Can you work these out from the model? Positions are in its coordinate system, mm. A direction names the side the tool comes from. Coordinates: 2 decimals unless noted, no trailing zeros. Write each loop counter-clockwise with the first axis right and the second up, starting at its lowest first coordinate (ties: lowest second). Pieces come first, ordered by that corner, then holes. Notation, with made-up numbers: (-33, 34) - (22, 34) arc R26 cw to (22, 51) - close; hole circle Ø7 at (1.25, 9). An arc over 180 degrees is marked (long way). Write each question's results on one line, items separated by ' | '. Start each with the question number.
```python
from build123d import *

# Parameters (mm, degrees)
SKETCH_1_W                = 120
SKETCH_1_H                = 20
EXTRUDE_1_DEPTH           = 4
HOLE_WIZARD_1_D           = 5.5
HOLE_WIZARD_1_CBORE_D     = 9.4
HOLE_WIZARD_1_CBORE_DEPTH = 5
HOLE_WIZARD_M5_2_D        = 4.2
SKETCH_6_W                = 45
SKETCH_6_H                = 10
CUT_EXTRUDE_1_DEPTH       = 62.351446601
CHAMFER_1_SIZE            = 10


with BuildPart() as part:
    # 草图1 → 凸台-拉伸1 (new, symmetric)
    with BuildSketch(Plane.XY):
        Rectangle(SKETCH_1_W, SKETCH_1_H)
    extrude(amount=EXTRUDE_1_DEPTH, both=True)

    # 打孔尺寸根据内六角圆柱头螺钉的类型1 (through all)
    with Locations(Plane(origin=(-5.332284739, -2.419582529, 4), x_dir=(1, 0, 0), z_dir=(0, 0, 1))):
        with Locations((-44.667715261, 7.419582529), (55.332284739, 7.419582529), (5.332284739, 7.419582529)):
            CounterBoreHole(HOLE_WIZARD_1_D / 2, HOLE_WIZARD_1_CBORE_D / 2, HOLE_WIZARD_1_CBORE_DEPTH)

    # M5 螺纹孔2 (through all)
    with Locations(Plane.XY.offset(4)):
        with Locations((-28.5, -5), (28.5, -5)):
            Hole(HOLE_WIZARD_M5_2_D / 2)

    # 草图6 → 切除-拉伸1 (cut, through all)
    with BuildSketch(Plane.XY.offset(4)):
        with Locations((0, -5)):
            Rectangle(SKETCH_6_W, SKETCH_6_H)
    extrude(amount=-CUT_EXTRUDE_1_DEPTH, mode=Mode.SUBTRACT)

    # 倒角1
    chamfer_1_edges = [part.edges().sort_by_distance(p)[0] for p in [
        (60, -10, 0),
        (-60, -10, 0),
    ]]
    chamfer(chamfer_1_edges, length=CHAMFER_1_SIZE)


solid = part.part
```
Q1. If we section it at C-C (y = 6): Please give me the cut outline in (x, z).
Q2. I'm going to push flat-ended pins straight in: pin 1 Ø1.5 at (y, z) = (-1, -2) entering from +X; pin 2 Ø4.5 at (x, y) = (-49.5, 5.5) entering from +Z; pin 3 Ø2.5 at (x, z) = (-11, -2) entering from -Y; pin 4 Ø11 at (x, y) = (-50, 5) entering from -Z. Where does each tip first touch, or does it pass through?
Q3. If we section it at D-D (x = 28.5): Please give me the cut outline in (y, z), then the cut area to 3 significant figures.
Q4. Thinking about a two-plate mould opening in X: for faces 1 (the face through (-36, -10, 0)), 2 (the face through (2.53, 8.96, 1.54)), 3 (the face through (60, 5, 0)), which applies, pulls with the +X half, pulls with the -X half, needs draft (parallel to the pull), parting line crosses it, or undercut?
Q5. If we section it at B-B (z = 0): Please give me the cut outline in (x, y), then the cut area to 3 significant figures.
Q6. If we section it at A-A (x = 0): Please give me the cut outline in (y, z).
Q7. I need wall thicknesses on line 1 along Y through (x, z) = (28.5, -0.5); line 2 along X through (y, z) = (-5.75, 2.5); line 3 along Y through (x, z) = (-50, -2.4). Which ranges of each line are inside material? Lowest first, please. Write a range as from..to.
Q8. For faces 4 (the face through (52.747, 5.121, -2.521)), 5 (the face through (-54.695, 5.207, 1.535)), 6 (the face through (-22.5, -5, 0)), which set-ups out of +Z, -Z, +X, -X, +Y, -Y let a thin tool reach every point of the face, with its end or its side?
Answer list:
1) outline: (-60, -4) - (-52.56, -4) - (-52.56, -1) - (-54.59, -1) - (-54.59, 4) - (-60, 4) - close; (-47.44, -4) - (-2.56, -4) - (-2.56, -1) - (-4.59, -1) - (-4.59, 4) - (-45.41, 4) - (-45.41, -1) - (-47.44, -1) - close; (2.56, -4) - (47.44, -4) - (47.44, -1) - (45.41, -1) - (45.41, 4) - (4.59, 4) - (4.59, -1) - (2.56, -1) - close; (52.56, -4) - (60, -4) - (60, 4) - (54.59, 4) - (54.59, -1) - (52.56, -1) - close
2) pin 1: stops at x = 59.75 | pin 2: stops at z = -1 | pin 3: stops at y = 0 | pin 4: stops at z = -4
3) outline: (-10, -4) - (-7.1, -4) - (-7.1, 4) - (-10, 4) - close; (-2.9, -4) - (10, -4) - (10, 4) - (-2.9, 4) - close | area: 126 mm2
4) face 1: needs draft | face 2: undercut | face 3: pulls with the +X half
5) outline: (-60, 0) - (-50, -10) - (-22.5, -10) - (-22.5, 0) - (22.5, 0) - (22.5, -10) - (50, -10) - (60, 0) - (60, 10) - (-60, 10) - close; hole circle Ø9.4 at (-50, 5); hole circle Ø4.2 at (-28.5, -5); hole circle Ø9.4 at (0, 5); hole circle Ø4.2 at (28.5, -5); hole circle Ø9.4 at (50, 5) | area: 1,610 mm2
6) outline: (0, -4) - (2.25, -4) - (2.25, -1) - (0.3, -1) - (0.3, 4) - (0, 4) - close; (7.75, -4) - (10, -4) - (10, 4) - (9.7, 4) - (9.7, -1) - (7.75, -1) - close
7) line 1: y = -10..-7.1, -2.9..10 | line 2: x = -54.25..-30.46, -26.54..-22.5, 22.5..26.54, 30.46..54.25 | line 3: y = -10..2.25, 7.75..10
8) face 4: +Z, -Z | face 5: +Z | face 6: +Z, -Z, -Y
